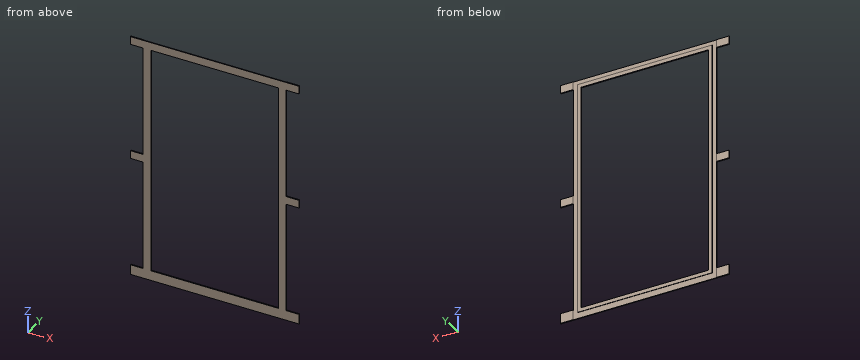
from build123d import *

# Parameters (mm, degrees)
SKETCH1_W           = 655
SKETCH1_H           = 1150
BOSS_EXTRUDE1_DEPTH = 6
SKETCH2_W           = 739
SKETCH2_H           = 1260
SKETCH2_W_2         = 693
SKETCH2_H_2         = 1188
CUT_EXTRUDE1_DEPTH  = 2


with BuildPart() as part:
    # Sketch1 → Boss-Extrude1 (new body)
    with BuildSketch(Plane(origin=(0, 0, 0), x_dir=(1, 0, 0), z_dir=(0, 1, 0))):
        Polygon((-433.5, 620), (433.5, 620), (433.5, 570), (367.5, 570), (367.5, 15), (433.5, 15), (433.5, -25), (367.5, -25), (367.5, -580), (433.5, -580), (433.5, -620), (-433.5, -620), (-433.5, -580), (-367.5, -580), (-367.5, -25), (-433.5, -25), (-433.5, 15), (-367.5, 15), (-367.5, 570), (-433.5, 570), align=None)
        with Locations((0, -5)):
            Rectangle(SKETCH1_W, SKETCH1_H, mode=Mode.SUBTRACT)
    extrude(amount=BOSS_EXTRUDE1_DEPTH)

    # Sketch2 → Cut-Extrude1 (cut)
    with BuildSketch(Plane(origin=(0, 6, 0), x_dir=(1, 0, 0), z_dir=(0, 1, 0))):
        Rectangle(SKETCH2_W, SKETCH2_H)
        with Locations((0, -5)):
            Rectangle(SKETCH2_W_2, SKETCH2_H_2, mode=Mode.SUBTRACT)
    extrude(amount=-CUT_EXTRUDE1_DEPTH, mode=Mode.SUBTRACT)


solid = part.part
Check sheet for the modelled part. Datum: model origin and axes. Units: mm. Give positions to 0.01 mm unless a question says otherwise; leave off trailing zeros. Write each loop counter-clockwise with the first axis right and the second up, starting at its lowest first coordinate (ties: lowest second). Pieces come first, ordered by that corner, then holes. Notation, with made-up numbers: (-7, -36.5) -> (51, -36.5) arc R21 ccw to (51, -31.5) -> close; hole circle Ø8 at (44.25, 8.5). An arc over 180 degrees is marked (long way). One line per item, written item: value. Start each with the question number.
Item 1: Section check B-B on x = 120. Record the cut outline in (y, z).
Item 2: Section check C-C on y = 2.6. Record the cut outline in (x, z).
Item 3: Gauge pin test, flat ends, axial feed: pin 1 (3 mm diameter, centred on y = 1.5, z = 384, fed in from +X); pin 2 (2 mm diameter, centred on y = 1.5, z = 238.5, fed in from -X); pin 3 (0.6 mm diameter, centred on y = 4.5, z = 50, fed in from -X). Record the tip position at first contact, or that the pin passes through.
Item 4: Section check A-A on z = 77. Record the cut outline in (x, y).
Item 5: Material ranges on probe 1 along Z at (x, y) = (-16, 2.6); probe 2 along X at (y, z) = (4.1, -557); probe 3 along Z at (x, y) = (148, 5.75), recorded low to high. Write a range as from..to.
Results list:
1. outline: (0, -620) -> (4, -620) -> (4, -589) -> (6, -589) -> (6, -570) -> (0, -570) -> close; (0, 580) -> (6, 580) -> (6, 599) -> (4, 599) -> (4, 620) -> (0, 620) -> close
2. outline: (-433.5, -620) -> (433.5, -620) -> (433.5, -570) -> (367.5, -570) -> (367.5, -15) -> (433.5, -15) -> (433.5, 25) -> (367.5, 25) -> (367.5, 580) -> (433.5, 580) -> (433.5, 620) -> (-433.5, 620) -> (-433.5, 580) -> (-367.5, 580) -> (-367.5, 25) -> (-433.5, 25) -> (-433.5, -15) -> (-367.5, -15) -> (-367.5, -570) -> (-433.5, -570) -> close; hole (-327.5, -570) -> (327.5, -570) -> (327.5, 580) -> (-327.5, 580) -> close
3. pin 1: x = 367.5
3. pin 2: x = -367.5
3. pin 3: x = -346.5
4. outline: (-367.5, 0) -> (-327.5, 0) -> (-327.5, 6) -> (-346.5, 6) -> (-346.5, 4) -> (-367.5, 4) -> close; (327.5, 0) -> (367.5, 0) -> (367.5, 4) -> (346.5, 4) -> (346.5, 6) -> (327.5, 6) -> close
5. probe 1: -620..-570, 580..620
5. probe 2: -346.5..-327.5, 327.5..346.5
5. probe 3: -589..-570, 580..599
